Design review of the part built by this model. Coordinates are the model's own, in mm. A direction names the side the tool comes from. Give positions to 0.01 mm unless a question says otherwise; leave off trailing zeros. Order: outer loops, then holes, each group sorted by start corner. A loop starts at its lowest first (then second) coordinate and runs counter-clockwise, first axis right, second up. Notation, with made-up numbers: (4, 63) -> (39, 63) arc R21 ccw to (39, 79) -> close; hole circle Ø8 at (11.5, 4). An arc over 180 degrees is marked (long way). One line per item, written item: value.
from build123d import *

# Parameters (mm, degrees)
SKETCH1_W                    = 53.808
SKETCH1_H                    = 16
BOSS_EXTRUDE1_DEPTH          = 1.4986
CONVERT_SOLID1_OUTLINE_W     = 53.808
CONVERT_SOLID1_OUTLINE_H     = 16
CONVERT_SOLID1_DEPTH         = 0.1316
EDGE_FLANGE1_STRIP_W         = 8.168
EDGE_FLANGE1_STRIP_H         = 1.367
EDGE_FLANGE1_STRIP_CUT_DEPTH = 53.808
EDGE_FLANGE1_DEPTH           = 53.808
M3_CLEARANCE_HOLE1_D         = 3.4


# Read off the part's stored shape, not the designer's step: Convert-Solid1
# Sheet-metal steps are written as plain solids
with BuildPart() as part:
    # Sketch1 → Boss-Extrude1 (new body)
    with BuildSketch(Plane.XY):
        with Locations((-41.271079995, -85.427168175)):
            Rectangle(SKETCH1_W, SKETCH1_H)
    extrude(amount=BOSS_EXTRUDE1_DEPTH)

    # Convert-Solid1 outline → Convert-Solid1 (cut)
    with BuildSketch(Plane.XY):
        with Locations((-41.271079995, -85.427168175)):
            Rectangle(CONVERT_SOLID1_OUTLINE_W, CONVERT_SOLID1_OUTLINE_H)
    extrude(amount=CONVERT_SOLID1_DEPTH, mode=Mode.SUBTRACT)

    # Edge-Flange1 strip (across the edge) → Edge-Flange1 strip cut (cut)
    with BuildSketch(Plane(origin=(-14.367079995, -93.427168175, 0.1316), x_dir=(0, 1, 0), z_dir=(-1, 0, 0))):
        with Locations((-2.734, -0.6835)):
            Rectangle(EDGE_FLANGE1_STRIP_W, EDGE_FLANGE1_STRIP_H)
    extrude(amount=EDGE_FLANGE1_STRIP_CUT_DEPTH, mode=Mode.SUBTRACT)

    # Edge-Flange1 section (across the edge) → Edge-Flange1 (add)
    with BuildSketch(Plane(origin=(-14.367079995, -93.427168175, 0.1316), x_dir=(0, 1, 0), z_dir=(-1, 0, 0))):
        with BuildLine():
            Line((-1.367, 1.35), (-1.367, 4.133))
            Line((-1.367, 4.133), (0, 4.133))
            Line((0, 4.133), (0, 1.35))
            ThreePointArc((0, 1.35), (0.395405845, 0.395405845), (1.35, 0))
            Line((1.35, 0), (1.35, -1.367))
            ThreePointArc((1.35, -1.367), (-0.571209124, -0.571209124), (-1.367, 1.35))
        make_face()
    extrude(amount=EDGE_FLANGE1_DEPTH)

    # M3 Clearance Hole1 (through all)
    with Locations(Plane(origin=(0, 0, 0.1316), x_dir=(-1, 0, 0), z_dir=(0, 0, -1))):
        with Locations((19.367079995, -81.427168175), (19.367079995, -88.427168175), (63.175079995, -88.427168175), (63.175079995, -81.427168175), (41.271079995, -88.427168175), (41.271079995, -81.427168175)):
            Hole(M3_CLEARANCE_HOLE1_D / 2)


solid = part.part
Item 1: Machinability: for faces 4 (the cylindrical face through (-40.36, -79.99, 0.82)), 5 (the flat face through (-41, -93.427, -3)), which of the approach directions +Z, -Z, +X, -X, +Y, -Y give a long, thin tool a straight path to every point of the face, cutting with its end or side? Answer none if there is none.
Returned:
face 4: +Z, -Z
face 5: -Z, +X, -X, +Y
Item 2: Draft analysis for pull direction Y (two halves, no side actions). For faces 1 (the flat face through (-68.175, -87.4, 0.4)), 2 (the flat face through (-41, -94.794, -3)), 3 (the cylindrical face through (-40.36, -86.99, 0.82)), state which applies: pulls with the +Y half, pulls with the -Y half, needs draft (parallel to the pull), parting line crosses it, or undercut.
Returned:
face 1: needs draft
face 2: pulls with the -Y half
face 3: undercut
Item 3: Add section A-A on x = -29. Give the boundary of the cut face in (y, z), plus the area to 3 significant figures.
Returned:
outline: (-94.79, -4) -> (-93.43, -4) -> (-93.43, -1.22) arc R1.35 cw to (-92.08, 0.13) -> (-77.43, 0.13) -> (-77.43, 1.5) -> (-92.08, 1.5) arc R2.72 ccw to (-94.79, -1.22) -> close
area: 28.2 mm²
Item 4: To check wall thickness, follow line 1 along X through (y, z) = (-88, 0.9); line 2 along Z through (x, y) = (-47.5, -82.75); line 3 along Y through (x, z) = (-38, -3.6). State the ranges of each line that lie inside material, in increasing order. Write a range as from..to.
Returned:
line 1: -68.18..-64.82, -61.53..-42.92, -39.63..-21.01, -17.72..-14.37
line 2: 0.13..1.5
line 3: -94.79..-93.43
Item 5: Add section C-C on z = -3. Give the boundary of the cut face in (x, y), plus the area to 3 significant figures.
Returned:
outline: (-68.18, -94.79) -> (-14.37, -94.79) -> (-14.37, -93.43) -> (-68.18, -93.43) -> close
area: 73.6 mm²
Item 6: Add section D-D on y = -87.25. Give the boundary of the cut face in (x, z).
Returned:
outline: (-68.18, 0.13) -> (-64.4, 0.13) -> (-64.4, 1.5) -> (-68.18, 1.5) -> close; (-61.95, 0.13) -> (-42.5, 0.13) -> (-42.5, 1.5) -> (-61.95, 1.5) -> close; (-40.04, 0.13) -> (-20.59, 0.13) -> (-20.59, 1.5) -> (-40.04, 1.5) -> close; (-18.14, 0.13) -> (-14.37, 0.13) -> (-14.37, 1.5) -> (-18.14, 1.5) -> close
Item 7: Clearance check with flat-ended pins moving along their axes: P1, Ø1.5, axis at x = -59, y = -82.5, coming from the -Z side; P2, Ø1.4, axis at x = -47, z = -3, coming from the +Y side. State where each tip first meets the part, or that it passes through.
Returned:
P1: z = 0.13
P2: y = -93.43
Item 8: Add section B-B on y = -80.75. Give the boundary of the cut face in (x, z), plus the area to 3 significant figures.
Returned:
outline: (-68.18, 0.13) -> (-64.73, 0.13) -> (-64.73, 1.5) -> (-68.18, 1.5) -> close; (-61.62, 0.13) -> (-42.83, 0.13) -> (-42.83, 1.5) -> (-61.62, 1.5) -> close; (-39.71, 0.13) -> (-20.93, 0.13) -> (-20.93, 1.5) -> (-39.71, 1.5) -> close; (-17.81, 0.13) -> (-14.37, 0.13) -> (-14.37, 1.5) -> (-17.81, 1.5) -> close
area: 60.8 mm²
